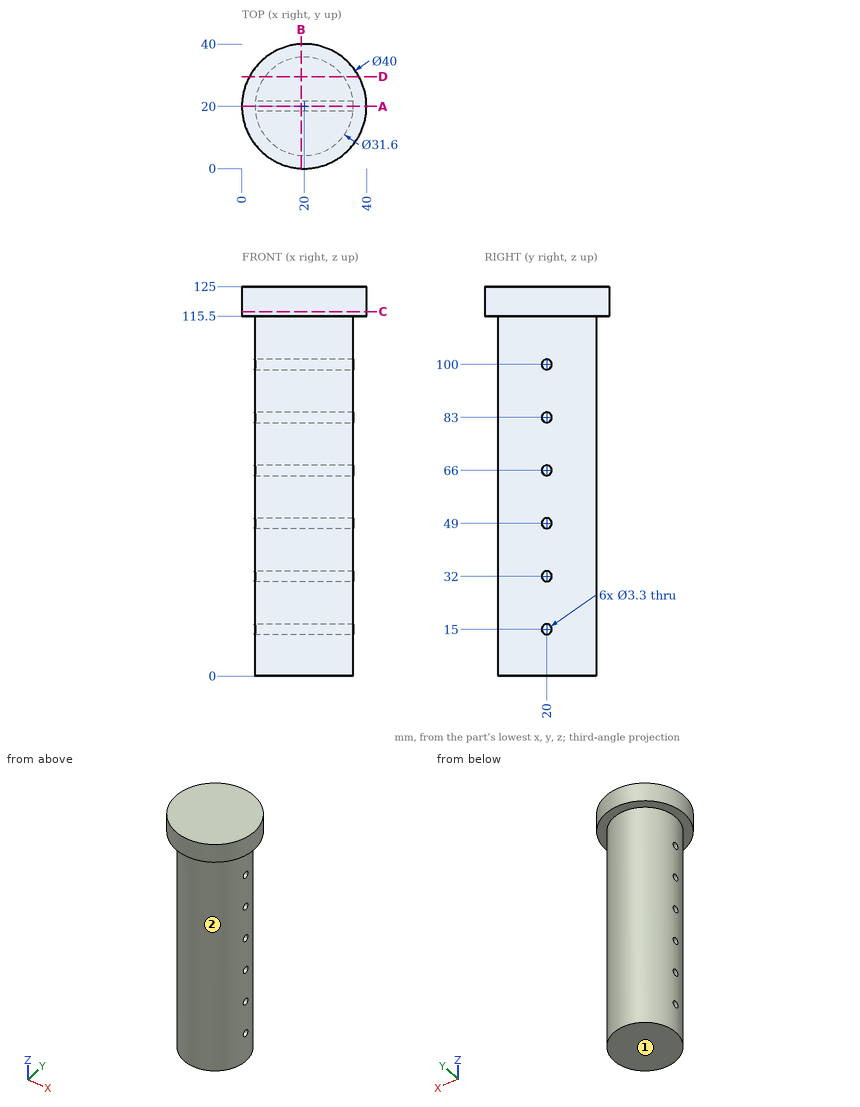
Geometry check sheet. Reference: drawing and pictorial views, mm from the part's lowest x, y, z. A direction names the side the tool comes from. Coordinates: 2 decimals unless noted, no trailing zeros. Order: outer loops, then holes, each group sorted by start corner. A loop starts at its lowest first (then second) coordinate and runs counter-clockwise, first axis right, second up.
Item 1: Section check A-A, the plane y = 20. Give the number of separate pieces and of enclosed holes in the cut face, then the cut area to 3 significant figures.
Filled in:
separate pieces: 7
enclosed holes: 0
area: 3,400 mm2
Item 2: Depth check by flat-ended pin: pin 1 (5 mm diameter, centred on x = 9.5, z = 107.5, fed in from -Y) (3 decimals); pin 2 (4 mm diameter, centred on y = 20, z = 100, fed in from +X); pin 3 (4 mm diameter, centred on y = 32.5, z = 45, fed in from -X). Enter the tip coordinate at first touch or a pass-through.
Filled in:
pin 1: stops at y = 6.375
pin 2: stops at x = 35.8
pin 3: stops at x = 8.19
Item 3: Material ranges on L1, parallel to Z at x = 8.5, y = 7; L2, parallel to Y at x = 15.5, z = 15; L3, parallel to X at y = 20, z = 23.5, recorded low to high.
Filled in:
L1: z = 115.5 to 125
L2: y = 4.85 to 18.35, 21.65 to 35.15
L3: x = 4.2 to 35.8
Item 4: Access from +Z, -Z, +X, -X, +Y, -Y to the whole of each face (thin tool, end or side, straight path). Record for the marked faces 1 and 2.
Filled in:
face 1: -Z, +X, -X, +Y, -Y
face 2: -Z
Item 5: Section check C-C, the plane z = 117. Enter the section's corners in (x, y), then the cut area to 3 significant figures.
Filled in:
outline: circle Ø40 at (20, 20)
area: 1,260 mm2
Item 6: Section check B-B, the plane x = 19. Enter the section's corners in (y, z), then the cut area to 3 significant figures.
Filled in:
outline: (0.03, 115.5) - (4.23, 115.5) - (4.23, 0) - (35.77, 0) - (35.77, 115.5) - (39.97, 115.5) - (39.97, 125) - (0.03, 125) - close; hole circle Ø3.3 at (20, 15); hole circle Ø3.3 at (20, 32); hole circle Ø3.3 at (20, 49); hole circle Ø3.3 at (20, 66); hole circle Ø3.3 at (20, 83); hole circle Ø3.3 at (20, 100)
area: 3,970 mm2
Item 7: Section check D-D, the plane y = 29.5. Enter the section's corners in (x, z).
Filled in:
outline: (2.4, 115.5) - (7.38, 115.5) - (7.38, 0) - (32.62, 0) - (32.62, 115.5) - (37.6, 115.5) - (37.6, 125) - (2.4, 125) - close
